```python
from build123d import *

# Parameters (mm, degrees)
SKETCH_1_R           = 1.625
EXTRUDE_1_DEPTH      = 4
SKETCH_2_W           = 30
SKETCH_2_H           = 11
EXTRUDE_2_DEPTH      = 4
SKETCH_3_W           = 30
SKETCH_3_H           = 24
EXTRUDE_3_DEPTH      = 4
EXTRUDE_4_DEPTH      = 30
SKETCH_5_W           = 4
SKETCH_5_H           = 23.7
EXTRUDE_5_DEPTH      = 30
SKETCH_6_W           = 30.00005
SKETCH_6_H           = 54.7
SKETCH_6_R           = 5.15
EXTRUDE_6_DEPTH      = 4
CUT_EXTRUDE_1_REACH  = 108.907
SKETCH_8_RX          = 7
SKETCH_8_RY          = 6
FILLET_START         = -32
FILLET_2_DEPTH       = 6
FILLET_3_R           = 15
EXTRUDE_8_DEPTH      = 4
EXTRUDE_8_DEPTH_BACK = 4
EXTRUDE_9_DEPTH      = 4
EXTRUDE_9_DEPTH_BACK = 4
SKETCH_13_R          = 0.5
CUT_EXTRUDE_2_DEPTH  = 20
SKETCH_14_W          = 4
SKETCH_14_H          = 8
CUT_EXTRUDE_3_DEPTH  = 10


with BuildPart() as part:
    # Эскиз1 → Бобышка-Вытянуть1 (new body)
    with BuildSketch(Plane(origin=(0, 0, 0), x_dir=(1, 0, 0), z_dir=(0, 1, 0))):
        Polygon((-10, 0), (10, 0), (10, 10), (15, 10), (15, 25.3), (-15, 25.3), (-15, 10), (-10, 10), align=None)
        with Locations(Location((-6, 15, 0), (0, 0, 270))):
            Circle(SKETCH_1_R, mode=Mode.SUBTRACT)
        with Locations(Location((0, 6, 0), (0, 0, 270))):
            Circle(SKETCH_1_R, mode=Mode.SUBTRACT)
        with Locations(Location((6, 15, 0), (0, 0, 90))):
            Circle(SKETCH_1_R, mode=Mode.SUBTRACT)
    extrude(amount=EXTRUDE_1_DEPTH)

    # Эскиз2 → Бобышка-Вытянуть2 (add)
    with BuildSketch(Plane(origin=(0, 0, -25.3), x_dir=(-1, 0, 0), z_dir=(0, 0, -1))):
        with Locations((0, -1.5)):
            Rectangle(SKETCH_2_W, SKETCH_2_H)
    extrude(amount=EXTRUDE_2_DEPTH)

    # Эскиз3 → Бобышка-Вытянуть3 (add)
    with BuildSketch(Plane.XZ.offset(7)):
        with Locations((0, -37.3)):
            Rectangle(SKETCH_3_W, SKETCH_3_H)
    extrude(amount=-EXTRUDE_3_DEPTH)

    # Эскиз4 → Бобышка-Вытянуть4 (add, through all)
    with BuildSketch(Plane.ZY.offset(15)):
        Polygon((-29.3, 4), (-29.3, -3), (-49.3, -3), align=None)
    extrude(amount=-EXTRUDE_4_DEPTH)

    # Эскиз5 → Бобышка-Вытянуть5 (add, through all)
    with BuildSketch(Plane(origin=(15, 0, 0), x_dir=(0, 0, -1), z_dir=(1, 0, 0))):
        with Locations((47.3, -18.85)):
            Rectangle(SKETCH_5_W, SKETCH_5_H)
    extrude(amount=-EXTRUDE_5_DEPTH)

    # Эскиз6 → Бобышка-Вытянуть6 (add)
    with BuildSketch(Plane.XZ.offset(30.7)):
        with Locations((-2.5e-05, -72.65)):
            Rectangle(SKETCH_6_W, SKETCH_6_H)
        with Locations(Location((-2.5e-05, -84, 0), (0, 0, 270))):
            Circle(SKETCH_6_R, mode=Mode.SUBTRACT)
    extrude(amount=-EXTRUDE_6_DEPTH)

    # Эскиз8 → Вырез-Вытянуть1 (cut, up to next)
    with BuildSketch(Plane.XZ.offset(30.7), mode=Mode.PRIVATE) as cut_extrude_1_sk1:
        with Locations(Location((15, -65.3), (0, 0, -90))):
            Ellipse(SKETCH_8_RX, SKETCH_8_RY)
    cut_extrude_1_tool1 = extrude(cut_extrude_1_sk1.sketch, amount=-CUT_EXTRUDE_1_REACH, mode=Mode.PRIVATE) & part.part
    # Эскиз8 → Вырез-Вытянуть1 (cut, up to next)
    with BuildSketch(Plane.XZ.offset(30.7), mode=Mode.PRIVATE) as cut_extrude_1_sk2:
        with Locations(Location((-15.000018282, -65.299986289), (0, 0, -90.000052373))):
            Ellipse(SKETCH_8_RX, SKETCH_8_RY)
    cut_extrude_1_tool2 = extrude(cut_extrude_1_sk2.sketch, amount=-CUT_EXTRUDE_1_REACH, mode=Mode.PRIVATE) & part.part
    add(cut_extrude_1_tool1.solids().sort_by_distance((15, -30.7, -65.3))[0], mode=Mode.SUBTRACT)
    add(cut_extrude_1_tool2.solids().sort_by_distance((-15.000018, -30.7, -65.299986))[0], mode=Mode.SUBTRACT)

    # Скругление2: read off the stored shape, not the designer's step
    # Скругление2 outline → Скругление2 (cut)
    with BuildSketch(Plane(origin=(0, 0, 0), x_dir=(1, 0, 0), z_dir=(0, 1, 0)).offset(FILLET_START)):
        with BuildLine():
            Line((15, 72.3), (15, 73.218180859))
            ThreePointArc((15, 73.218180859), (14.762336304, 72.570999772), (14.162313281, 72.231441583))
            add(Edge.make_bspline(
                [(14.162313281, 72.231441583), (14.579095458, 72.3), (15, 72.3)],
                knots=[6.131749827, 6.131749827, 6.131749827, 6.283185307, 6.283185307, 6.283185307], degree=2, weights=[0.948970652, 0.971763096, 1]))
        make_face()
        with BuildLine():
            add(Edge.make_bspline(
                [(15, 58.3), (14.579095458, 58.3), (14.162313281, 58.368558417)],
                knots=[3.141592654, 3.141592654, 3.141592654, 3.293028134, 3.293028134, 3.293028134], degree=2, weights=[1, 0.971763096, 0.948970652]))
            ThreePointArc((14.162313281, 58.368558417), (14.762336304, 58.029000228), (15, 57.381819141))
            Line((15, 57.381819141), (15, 58.3))
        make_face()
        with BuildLine():
            add(Edge.make_bspline(
                [(-15.00005, 72.299986289), (-14.579143154, 72.299988746), (-14.162358429, 72.231432015)],
                knots=[6.283181087, 6.283181087, 6.283181087, 6.434617466, 6.434617466, 6.434617466], degree=2, weights=[1, 0.971762843, 0.948970209]))
            ThreePointArc((-14.162358429, 72.231432015), (-14.762384713, 72.570989127), (-15.00005, 73.218172089))
            Line((-15.00005, 73.218172089), (-15.00005, 72.299986289))
        make_face()
        with BuildLine():
            ThreePointArc((-15.00005, 57.381799936), (-14.762384538, 58.028983103), (-14.162357897, 58.368540098))
            add(Edge.make_bspline(
                [(-14.162357897, 58.368540098), (-14.579142884, 58.299983554), (-15.00005, 58.299986289)],
                knots=[9.27334784, 9.27334784, 9.27334784, 9.424784314, 9.424784314, 9.424784314], degree=2, weights=[0.948970181, 0.971762826, 1]))
            Line((-15.00005, 58.299986289), (-15.00005, 57.381799936))
        make_face()
    extrude(amount=FILLET_2_DEPTH, mode=Mode.SUBTRACT)

    # Скругление3
    fillet_3_edges = [part.edges().sort_by_distance(p)[0] for p in [
        (-15.00005, -28.7, -100),
        (15, -28.7, -100),
    ]]
    fillet(fillet_3_edges, radius=FILLET_3_R)

    # Эскиз10 → Бобышка-Вытянуть8 (add, two sides: drawn at the far end of the back side and taken through both)
    with BuildSketch(Plane.ZY.offset(2.5e-05).offset(-EXTRUDE_8_DEPTH_BACK)):
        Polygon((-49.3, -26.7), (-73.3, -26.7), (-49.3, -3), align=None)
    extrude(amount=EXTRUDE_8_DEPTH + EXTRUDE_8_DEPTH_BACK)

    # Эскиз11 → Бобышка-Вытянуть9 (add, two sides: drawn at the far end of the back side and taken through both)
    with BuildSketch(Plane.ZY.offset(2.5e-05).offset(-EXTRUDE_9_DEPTH_BACK)):
        Polygon((-31.3, -7), (-45.3, -7), (-45.3, -30.7), align=None)
    extrude(amount=EXTRUDE_9_DEPTH + EXTRUDE_9_DEPTH_BACK)

    # Эскиз13 → Вырез-Вытянуть2 (cut)
    with BuildSketch(Plane.XZ.offset(30.7)):
        with Locations(Location((-1.0754e-05, -76.47, 0), (0, 0, 270))):
            Circle(SKETCH_13_R)
        with Locations(Location((-1.2125e-05, -73.47, 0), (0, 0, 270))):
            Circle(SKETCH_13_R)
        with Locations(Location((-1.3496e-05, -70.47, 0), (0, 0, 270))):
            Circle(SKETCH_13_R)
        with Locations(Location((-1.4867e-05, -67.47, 0), (0, 0, 270))):
            Circle(SKETCH_13_R)
        with Locations(Location((-3.871e-06, -91.53, 0), (0, 0, 270))):
            Circle(SKETCH_13_R)
    extrude(amount=-CUT_EXTRUDE_2_DEPTH, mode=Mode.SUBTRACT)

    # Эскиз14 → Вырез-Вытянуть3 (cut)
    with BuildSketch(Plane(origin=(0, -26.7, 0), x_dir=(1, 0, 0), z_dir=(0, 1, 0))):
        with Locations((-2.5e-05, 69.3)):
            Rectangle(SKETCH_14_W, SKETCH_14_H)
    extrude(amount=CUT_EXTRUDE_3_DEPTH, mode=Mode.SUBTRACT)


solid = part.part
```
Read the model definition and answer for the solid it produces. Units are mm, in the model's axes. A direction names the side the tool comes from. Give positions to 0.01 mm unless a question says otherwise; leave off trailing zeros. Order: outer loops, then holes, each group sorted by start corner. A loop starts at its lowest first (then second) coordinate and runs counter-clockwise, first axis right, second up.
(1) Straight lines are drawn through the part: L1, parallel to X at y = 2, z = -15 (3 decimals); L2, parallel to Y at x = 10, z = -81.5; L3, parallel to Y at x = 6.5, z = -5. For each, find the intervals that lie inside material, in ascending order.
(2) Find section A-A (z = -84). Give the vertices of the cut face in (x, y).
(3) For a pull along X with two mould halves and no side action, classify faces 1 (the flat face through (15, -29, -79)), 2 (the flat face through (-10, 2, -5)), 3 (the cylindrical face through (1.55, -28.73, -88.91)) as released by +X, released by -X, zero draft, split by the parting line, or undercut.
(4) Given pin 1 (1.2 mm diameter, centred on y = 1.5, z = -3.5, fed in from -X); pin 2 (5.5 mm diameter, centred on x = 3.5, y = -4, fed in from +Z); pin 3 (4 mm diameter, centred on x = 6, z = -15, fed in from +Y); pin 4 (9 mm diameter, centred on x = -7, y = -10.5, fed in from -Z), each flat-ended and moving along its own axis, determine where each tip first touches the part or whether it passes through.
(5) Find section C-C (y = -13.5). Give the vertices of the cut face in (x, z).
(6) Find section B-B (y = 1.5). Give the vertices of the cut face in (x, z) (3 decimals).
(7) For faces 4 (the flat face through (4, -16, -40)), 5 (the flat face through (0, -26.7, -78)), 6 (the flat face through (4, -20, -56)), 7 (the flat face through (10, 2, -5)), determine the directions among +Z, -Z, +X, -X, +Y, -Y from which every point of the face is accessible in a straight line to the end or side of a thin tool.
(8) Find section D-D (z = -36). Give the vertices of the cut face in (x, y) (3 decimals), plus the area to 3 significant figures.
Result sheet:
1. L1: x = -15 to -7.625, -4.375 to 4.375, 7.625 to 15
1. L2: y = -30.7 to -26.7
1. L3: y = 0 to 4
2. outline: (-15, -30.7) - (-5.15, -30.7) - (-5.15, -26.7) - (-15, -26.7) - close; (5.15, -30.7) - (15, -30.7) - (15, -26.7) - (5.15, -26.7) - close
3. face 1: released by +X
3. face 2: released by -X
3. face 3: undercut
4. pin 1: stops at x = -10
4. pin 2: stops at z = -25.3
4. pin 3: stops at y = 4
4. pin 4: stops at z = -60.29
5. outline: (-15, -49.3) - (-4, -49.3) - (-4, -59.93) - (4, -59.93) - (4, -49.3) - (15, -49.3) - (15, -45.3) - (4, -45.3) - (4, -35.14) - (-4, -35.14) - (-4, -45.3) - (-15, -45.3) - close
6. outline: (-15, -36.443) - (15, -36.443) - (15, -10) - (10, -10) - (10, 0) - (-10, 0) - (-10, -10) - (-15, -10) - close; hole circle Ø3.25 at (-6, -15); hole circle Ø3.25 at (0, -6); hole circle Ø3.25 at (6, -15)
7. face 4: +Z, +X, -Y
7. face 5: -Z, +Y
7. face 6: -Z, +X, +Y
7. face 7: +Z, +X, +Y, -Y
8. outline: (-15, -7) - (-4, -7) - (-4, -14.956) - (4, -14.956) - (4, -7) - (15, -7) - (15, 1.655) - (-15, 1.655) - close
8. area: 323 mm2
